Geometry: final body of the model. Coordinates: model frame, mm. A direction names the side the tool comes from. Round coordinates to 2 decimals unless told otherwise and drop trailing zeros. Loops run counter-clockwise (first coordinate to the right, second up) from the corner with the lowest first, then second, coordinate; pieces in that order, holes last. Notation, with made-up numbers: (69.25, 18) -> (114.25, 18) arc R19 cw to (114.25, 46) -> close; hole circle Ø2 at (72.25, 54). An arc over 180 degrees is marked (long way). Answer in a Markdown table with one row per item.
```python
from build123d import *

# Parameters (mm, degrees)
F0_W     = 135
F0_H     = 60
F1_DEPTH = 16
F2_W     = 1.12
F2_H     = 60
F3_DEPTH = 14
F4_R     = 2
F5_W     = 135
F5_H     = 12
F6_DEPTH = 8


with BuildPart() as f1:
    # F0 (on Top) → F1 (new body)
    with BuildSketch(Plane.XY):
        Rectangle(F0_W, F0_H)
    extrude(amount=F1_DEPTH)

    # F2 (on face) → F3 (cut)
    with BuildSketch(Plane.XY.offset(16)):
        Polygon((16.9943201199, 30), (15.1943201199, 30), (-67.5, -17.7435879817), (-67.5, -18.7828184662), align=None)
        Polygon((35.2673136497, 30), (33.0273136497, 30), (-67.5, -28.0394715965), (-67.5, -29.3327361995), align=None)
        with Locations((42.1117129004, 0)):
            Rectangle(F2_W, F2_H)
    extrude(amount=-F3_DEPTH, mode=Mode.SUBTRACT)

    # F4
    f4_edges = [f1.edges().sort_by_distance(p)[0] for p in [
        (-12.974144, -30, 16),
        (-67.5, 6.128206, 16),
        (67.5, 0, 16),
        (55.085856, -30, 16),
    ]]
    fillet(f4_edges, radius=F4_R)

    # F5 (on face) → F6 (join)
    with BuildSketch(Plane(origin=(0, 0, 0), x_dir=(1, 0, 0), z_dir=(0, 0, -1))):
        with Locations((0, 24)):
            Rectangle(F5_W, F5_H)
    extrude(amount=F6_DEPTH)


solid = f1.part
```
Item 1: First-contact query: P1, Ø1.2, axis at x = 42.5, y = 2, coming from the +Z side; P2, Ø4, axis at x = 20, y = 2.5, coming from the -Z side; P3, Ø4, axis at x = 1, z = -5, coming from the +Y side. Flat tips, straight axial feed; report the tip coordinate or a pass-through.
Ans:
| item | result |
|---|---|
| P1 | z = 16 |
| P2 | z = 0 |
| P3 | y = -18 |
Item 2: Section query D-D, the plane z = -3.5. Output: boundary loops of the cut face in (x, y), and give its area (3 significant figures).
Ans:
| item | result |
|---|---|
| outline | (-67.5, -30) -> (67.5, -30) -> (67.5, -18) -> (-67.5, -18) -> close |
| area | 1,620 mm2 |
Item 3: Mould query, pull axis Y, two halves, no side actions, for faces 1 (the flat face through (-1, -18, -4)), 2 (the flat face through (-16.53, 1.39, 9.1)), 3 (the flat face through (-1, 6, 0)). Classes: released by +Y, released by -Y, zero draft, split by the parting line, or undercut.
Ans:
| item | result |
|---|---|
| face 1 | released by +Y |
| face 2 | undercut |
| face 3 | zero draft |
Item 4: Set-up query: faces 4 (the flat face through (67.5, 0, 6)), 5 (the flat face through (-25.84, 5.27, 9.1)), 6 (the flat face through (42.672, 0, 9)). Return all of +Z, -Z, +X, -X, +Y, -Y with unobstructed straight access to the full face (end or side cutting, diameter ignored); none if empty.
Ans:
| item | result |
|---|---|
| face 4 | +Z, -Z, +X, +Y, -Y |
| face 5 | +Z |
| face 6 | +Z, +Y, -Y |
Item 5: Section query C-C, the plane x = 52. Output: boundary loops of the cut face in (y, z).
Ans:
| item | result |
|---|---|
| outline | (-30, -8) -> (-18, -8) -> (-18, 0) -> (30, 0) -> (30, 16) -> (-28, 16) arc R2 ccw to (-30, 14) -> close |
Item 6: Section query B-B, the plane y = 8. Output: boundary loops of the cut face in (x, z), and give its area (3 significant figures).
Ans:
| item | result |
|---|---|
| outline | (-67.5, 0) -> (67.5, 0) -> (67.5, 14) arc R2 ccw to (65.5, 16) -> (42.67, 16) -> (42.67, 2) -> (41.55, 2) -> (41.55, 16) -> (-2.84, 16) -> (-2.84, 2) -> (-5.08, 2) -> (-5.08, 16) -> (-21.11, 16) -> (-21.11, 2) -> (-22.91, 2) -> (-22.91, 16) -> (-65.5, 16) arc R2 ccw to (-67.5, 14) -> close |
| area | 2,090 mm2 |
Item 7: Section query A-A, the plane z = 10.5. Output: boundary loops of the cut face in (x, y).
Ans:
| item | result |
|---|---|
| outline | (-67.5, -30) -> (41.55, -30) -> (41.55, 30) -> (35.27, 30) -> (-67.5, -29.33) -> close; (-67.5, -28.04) -> (33.03, 30) -> (16.99, 30) -> (-67.5, -18.78) -> close; (-67.5, -17.74) -> (15.19, 30) -> (-67.5, 30) -> close; (42.67, -30) -> (67.5, -30) -> (67.5, 30) -> (42.67, 30) -> close |
Item 8: Ray query, L1, parallel to Y at x = -11.5, z = 14.5; L2, parallel to Y at x = 10, z = 10.25; L3, parallel to X at y = -0.5, z = 9.75. Return the intervals inside material, ascending.
Ans:
| item | result |
|---|---|
| L1 | -29.94 to 3, 4.29 to 13.55, 14.59 to 30 |
| L2 | -30 to 15.41, 16.71 to 25.96, 27 to 30 |
| L3 | -67.5 to -37.63, -35.83 to -19.8, -17.56 to 41.55, 42.67 to 67.5 |
